Part model, mm, in its own coordinate system. A direction names the side the tool comes from. Give positions to 0.01 mm unless a question says otherwise; leave off trailing zeros. Write each loop counter-clockwise with the first axis right and the second up, starting at its lowest first coordinate (ties: lowest second). Pieces come first, ordered by that corner, then holes. Notation, with made-up numbers: M 78,-34.5 L 133,-34.5 A13 ccw 133,-20.5 Z; hole C -35,6.25 d1. An arc over 180 degrees is marked long. Answer as CSV lines item,"result". Start each with the question number.
Item 1: Pin check, flat tips, straight feed: pin 1 (1.2 mm diameter, centred on x = 6.5, z = 1.5, fed in from +Y); pin 2 (12 mm diameter, centred on x = -28.5, y = 21.5, fed in from -Z). Stop position of each tip, or through.
Item 2: Band-saw the part on D-D, the plane y = -11. List the corners of the cut face in (x, z).
Item 3: 3-axis set-ups, long thin cutter, end or side, ignore diameter. For faces 1 (the cylindrical face through (25.089, 17.065, 1.268)), 2 (the flat face through (0, -15, 1)), 3 (the cylindrical face through (-35.525, 4.254, 1.268)), 4 (the flat face through (46.45, -24.15, 1.23)): which of +Z, -Z, +X, -X, +Y, -Y reach the whole face in a straight line?
Item 4: Wall check: L1, parallel to X at y = 37.5, z = 2.2; L2, parallel to Y at x = -45.5, z = 1.9; L3, parallel to X at y = 29.5, z = 0.35. Give the ranges that are in metal, low to high. Write a range as from..to.
Item 5: Band-saw the part on C-C, the plane x = 50. List the corners of the cut face in (y, z).
Item 6: Band-saw the part on B-B, the plane x = -50. List the corners of the cut face in (y, z).
Item 7: Band-saw the part on A-A, the plane z = 0.9. List the corners of the cut face in (x, y).
Item 8: Two-plate mould, pull along Y, no slides. Class faces 5 (the cylindrical face through (24.899, -16.955, 1.268)), 6 (the flat face through (46.19, 23.7, 1.23)), 7 (the flat face through (-1, 1, 0)): +Y half, -Y half, draft (parallel to the pull), parting line (faces both ways), or undercut.
from build123d import *

# Parameters (mm, degrees)
F1_DEPTH = 2.5
F2_R     = 15


with BuildPart() as f1:
    # F0 (on Top) → F1 (new body)
    with BuildSketch(Plane.XY):
        with BuildLine():
            ThreePointArc((-44.547231, 46.839252), (-53.25, 48.930435), (-55.790366, 40.348025))
            Line((-55.790366, 40.348025), (-35, 4.338054))
            Line((-35, 4.338054), (-35, 0))
            Line((-35, 0), (-35, -4.338054))
            Line((-35, -4.338054), (-55.790366, -40.348025))
            ThreePointArc((-55.790366, -40.348025), (-53.25, -48.930435), (-44.547231, -46.839252))
            Line((-44.547231, -46.839252), (-26.164831, -15))
            Line((-26.164831, -15), (0, -15))
            Line((0, -15), (26.154701, -15))
            Line((26.154701, -15), (44.370835, -46.55127))
            ThreePointArc((44.370835, -46.55127), (53.25, -48.930435), (55.629165, -40.05127))
            Line((55.629165, -40.05127), (35, -4.320508))
            Line((35, -4.320508), (35, 0))
            Line((35, 0), (35, 4.320508))
            Line((35, 4.320508), (55.629165, 40.05127))
            ThreePointArc((55.629165, 40.05127), (53.25, 48.930435), (44.370835, 46.55127))
            Line((44.370835, 46.55127), (26.154701, 15))
            Line((26.154701, 15), (0, 15))
            Line((0, 15), (-26.164831, 15))
            Line((-26.164831, 15), (-44.547231, 46.839252))
        make_face()
    extrude(amount=F1_DEPTH)

    # F2
    f2_edges = [f1.edges().sort_by_distance(p)[0] for p in [
        (26.154701, 15, 1.25),
        (-26.164831, 15, 1.25),
        (26.154701, -15, 1.25),
        (-26.164831, -15, 1.25),
        (-35, -4.338054, 1.25),
        (-35, 4.338054, 1.25),
        (35, -4.320508, 1.25),
        (35, 4.320508, 1.25),
    ]]
    fillet(f2_edges, radius=F2_R)


solid = f1.part
Output:
1,pin 1,"y = 15"
1,pin 2,"z = 0"
2,outline,"M -38.85,0 L 38.86,0 L 38.86,2.5 L -38.85,2.5 Z"
3,face 1,"+Z, -Z, +Y"
3,face 2,"+Z, -Z, -Y"
3,face 3,"+Z, -Z, -X"
3,face 4,"+Z, -Z, +X"
4,L1,"-54.15..-39.16, 39.15..54.16"
4,L2,"-47.99..-22.52, 22.52..47.99"
4,L3,"-49.53..-34.54, 34.53..49.54"
5,outline,"M -49.8,0 L -30.3,0 L -30.3,2.5 L -49.8,2.5 Z; M 30.3,0 L 49.8,0 L 49.8,2.5 L 30.3,2.5 Z"
6,outline,"M -49.8,0 L -30.32,0 L -30.32,2.5 L -49.8,2.5 Z; M 30.32,0 L 49.8,0 L 49.8,2.5 L 30.32,2.5 Z"
7,outline,"M -55.79,-40.35 A6.5 ccw -44.55,-46.84 L -30.49,-22.5 A15 cw -17.5,-15 L 17.49,-15 A15 cw 30.48,-22.5 L 44.37,-46.55 A6.5 ccw 55.63,-40.05 L 37.01,-7.8 A15 cw 35,-0.3 L 35,0.3 A15 cw 37.01,7.8 L 55.63,40.05 A6.5 ccw 44.37,46.55 L 30.48,22.5 A15 cw 17.49,15 L -17.5,15 A15 cw -30.49,22.5 L -44.55,46.84 A6.5 ccw -55.79,40.35 L -37.01,7.82 A15 cw -35,0.32 L -35,-0.32 A15 cw -37.01,-7.82 Z"
8,face 5,"-Y half"
8,face 6,"undercut"
8,face 7,"draft"
